from build123d import *

# Parameters (mm, degrees)
SKETCH_1_W             = 47.4
SKETCH_1_H             = 36
EXTRUDE_1_DEPTH        = 78.5
FILLET_1_R             = 2
HOLE_WIZARD_M3_1_D     = 2.5
HOLE_WIZARD_M3_1_DEPTH = 4
HOLE_WIZARD_M3_1_TIP   = 0.751075774
SKETCH_4_R             = 9
CUT_EXTRUDE_1_DEPTH    = 2
SKETCH_5_R             = 6
EXTRUDE_2_DEPTH        = 8


with BuildPart() as part:
    # 草图1 → 凸台-拉伸1 (new, symmetric)
    with BuildSketch(Plane(origin=(0, 0, 0), x_dir=(0, 0, -1), z_dir=(1, 0, 0))):
        Rectangle(SKETCH_1_W, SKETCH_1_H)
    extrude(amount=EXTRUDE_1_DEPTH, both=True)

    # 圆角1
    fillet_1_edges = [part.edges().sort_by_distance(p)[0] for p in [
        (78.5, 0, 23.7),
        (78.5, -18, 0),
        (78.5, 0, -23.7),
        (-78.5, -18, 0),
        (-78.5, 0, 23.7),
        (-78.5, 18, 0),
        (-78.5, 0, -23.7),
        (78.5, 18, 0),
        (0, -18, -23.7),
        (0, -18, 23.7),
        (0, 18, 23.7),
        (0, 18, -23.7),
    ]]
    fillet(fillet_1_edges, radius=FILLET_1_R)

    # M3 螺纹孔1
    with Locations(Plane(origin=(0, 18, 41.7), x_dir=(1, 0, 0), z_dir=(0, 1, 0))):
        with Locations((-33, 43.1), (33, 43.1)):
            Hole(HOLE_WIZARD_M3_1_D / 2, depth=HOLE_WIZARD_M3_1_DEPTH)
            with Locations((0, 0, -(HOLE_WIZARD_M3_1_DEPTH + HOLE_WIZARD_M3_1_TIP / 2))):  # 118° drill point
                Cone(0, HOLE_WIZARD_M3_1_D / 2, HOLE_WIZARD_M3_1_TIP, mode=Mode.SUBTRACT)

    # 草图4 → 切除-拉伸1 (cut)
    with BuildSketch(Plane(origin=(0, 0, -23.7), x_dir=(-1, 0, 0), z_dir=(0, 0, -1))):
        with Locations((60, 0)):
            Circle(SKETCH_4_R)
        with Locations((-60, 0)):
            Circle(SKETCH_4_R)
    extrude(amount=-CUT_EXTRUDE_1_DEPTH, mode=Mode.SUBTRACT)

    # 草图5 → 凸台-拉伸2 (add)
    with BuildSketch(Plane.XY.offset(23.7)):
        with Locations(Location((0, 0, 0), (0, 0, 180))):
            Circle(SKETCH_5_R)
    extrude(amount=EXTRUDE_2_DEPTH)


solid = part.part
Verification items for the finished model (mm, model axes). A direction names the side the tool comes from. Coordinates: 2 decimals unless noted, no trailing zeros. Order: outer loops, then holes, each group sorted by start corner. A loop starts at its lowest first (then second) coordinate and runs counter-clockwise, first axis right, second up.
Item 1: Depth check by flat-ended pin: pin 1 (10 mm diameter, centred on x = 60.5, y = 12, fed in from +Z); pin 2 (9 mm diameter, centred on x = -62.5, y = 0, fed in from -Z). Enter the tip coordinate at first touch or a pass-through.
Filled in:
pin 1: stops at z = 23.7
pin 2: stops at z = -21.7
Item 2: Access from +Z, -Z, +X, -X, +Y, -Y to the whole of each face (thin tool, end or side, straight path). Record for faces 5 (the face through (78.5, 0, 0)), 6 (the face through (-60, 0, -21.7)).
Filled in:
face 5: +Z, -Z, +X, +Y, -Y
face 6: -Z
Item 3: Material ranges on L1, parallel to X at y = 17, z = -1; L2, parallel to Z at x = 71, y = -1; L3, parallel to Z at x = 53, y = -3, recorded low to high.
Filled in:
L1: x = -78.23 to -34.18, -31.82 to 31.82, 34.18 to 78.23
L2: z = -23.7 to 23.7
L3: z = -21.7 to 23.7
Item 4: Section check D-D, the plane x = -60. Enter the section's corners in (y, z), then the cut area to 3 significant figures.
Filled in:
outline: (-18, -21.7) arc R2 ccw to (-16, -23.7) - (-9, -23.7) - (-9, -21.7) - (9, -21.7) - (9, -23.7) - (16, -23.7) arc R2 ccw to (18, -21.7) - (18, 21.7) arc R2 ccw to (16, 23.7) - (-16, 23.7) arc R2 ccw to (-18, 21.7) - close
area: 1,670 mm2
Item 5: Section check A-A, the plane x = 0. Enter the section's corners in (y, z), then the cut area to 3 significant figures.
Filled in:
outline: (-18, -21.7) arc R2 ccw to (-16, -23.7) - (16, -23.7) arc R2 ccw to (18, -21.7) - (18, 21.7) arc R2 ccw to (16, 23.7) - (6, 23.7) - (6, 31.7) - (-6, 31.7) - (-6, 23.7) - (-16, 23.7) arc R2 ccw to (-18, 21.7) - close
area: 1,800 mm2
Item 6: Section check C-C, the plane x = 27. Enter the section's corners in (y, z), then the cut area to 3 significant figures.
Filled in:
outline: (-18, -21.7) arc R2 ccw to (-16, -23.7) - (16, -23.7) arc R2 ccw to (18, -21.7) - (18, 21.7) arc R2 ccw to (16, 23.7) - (-16, 23.7) arc R2 ccw to (-18, 21.7) - close
area: 1,700 mm2
Item 7: Release check for a two-part mould opening along Y. For faces 1 (the face through (1, -7, 23.7)), 2 (the face through (51.416, 2.703, -22.714)), 3 (the face through (-5.723, -1.802, 27.644)), 4 (the face through (60, 0, -21.7)) record: +Y half, -Y half, draft (parallel to the pull), parting line (faces both ways), or undercut.
Filled in:
face 1: draft
face 2: undercut
face 3: parting line
face 4: undercut
Item 8: Section check B-B, the plane y = 0. Enter the section's corners in (x, z).
Filled in:
outline: (-78.5, -21.7) arc R2 ccw to (-76.5, -23.7) - (-69, -23.7) - (-69, -21.7) - (-51, -21.7) - (-51, -23.7) - (51, -23.7) - (51, -21.7) - (69, -21.7) - (69, -23.7) - (76.5, -23.7) arc R2 ccw to (78.5, -21.7) - (78.5, 21.7) arc R2 ccw to (76.5, 23.7) - (6, 23.7) - (6, 31.7) - (-6, 31.7) - (-6, 23.7) - (-76.5, 23.7) arc R2 ccw to (-78.5, 21.7) - close
